from build123d import *

# Parameters (mm, degrees)
F0_W     = 250
F0_H     = 100
F1_DEPTH = 20
F2_W     = 50
F2_H     = 75
F2_W_2   = 44
F2_H_2   = 69
F3_DEPTH = 1200
F4_W     = 50
F4_H     = 75
F4_W_2   = 44
F4_H_2   = 69
F5_DEPTH = 837.2
F6_F1_R  = 1.5
F6_F2_R  = 1.5
F6_F3_R  = 1.5
F6_F4_R  = 1.4999


# Not quite as in the source:
# - a fillet or chamfer is up to 0.001 mm smaller than in the source, because OpenCascade refuses the exact size


with BuildPart() as f1:
    # F0 (on Top) → F1 (new body)
    with BuildSketch(Plane.XY):
        Rectangle(F0_W, F0_H)
    extrude(amount=F1_DEPTH)

    # F2 (on face) → F3 (join)
    with BuildSketch(Plane.XY.offset(20)):
        Rectangle(F2_W, F2_H)
        Rectangle(F2_W_2, F2_H_2, mode=Mode.SUBTRACT)
    extrude(amount=F3_DEPTH)

    # F4 (on face) → F5 (join)
    with BuildSketch(Plane.XZ.offset(37.5)):
        with Locations((0, 1257.5)):
            Rectangle(F4_W, F4_H)
        with Locations((0, 1257.5)):
            Rectangle(F4_W_2, F4_H_2, mode=Mode.SUBTRACT)
    extrude(amount=-F5_DEPTH)

    # F6: fillet of radius 1.5 on 44 edges, made by hand

    # F6_f1
    f6_f1_edges = [f1.edges().sort_by_distance(p)[0] for p in [
        (-22, -34.5, 620),
        (22, 34.5, 620),
        (22, -34.5, 620),
        (-22, 34.5, 620),
        (-22, 381.1, 1292),
        (22, 381.1, 1292),
        (0, 37.5, 1220),
        (22, 381.1, 1223),
        (-22, 381.1, 1223),
        (22, 0, 1220),
        (0, -34.5, 1220),
        (-22, 0, 1220),
        (0, 34.5, 1220),
        (0, 34.5, 20),
        (-22, 0, 20),
        (22, 0, 20),
        (0, -34.5, 20),
    ]]
    fillet(f6_f1_edges, radius=F6_F1_R)

    # F6_f2
    f6_f2_edges = [f1.edges().sort_by_distance(p)[0] for p in [
        (-25, -37.5, 657.5),
        (25, 37.5, 619.25),
        (25, -37.5, 657.5),
        (-25, 37.5, 619.25),
        (25, 381.1, 1295),
        (-25, 381.1, 1295),
        (0, -37.5, 1295),
        (125, -50, 10),
        (-125, -50, 10),
        (125, 50, 10),
        (0, -50, 0),
        (0, -50, 20),
        (0, 50, 20),
        (125, 0, 20),
        (-125, 0, 20),
        (-125, 50, 10),
        (0, 50, 0),
        (125, 0, 0),
        (-125, 0, 0),
        (-25, 37.9393398282, 1219.5606601718),
        (25, 37.9393398282, 1219.5606601718),
    ]]
    fillet(f6_f2_edges, radius=F6_F2_R)

    # F6_f3
    f6_f3_edges = [f1.edges().sort_by_distance(p)[0] for p in [
        (25, 0, 20),
        (-25, 0, 20),
        (0, -37.5, 20),
        (0, 37.5, 20),
        (24.5606601718, 37.0606601718, 20),
        (-24.5606601718, 37.0606601718, 20),
        (-24.5606601718, -37.0606601718, 20),
        (24.5606601718, -37.0606601718, 20),
    ]]
    fillet(f6_f3_edges, radius=F6_F3_R)

    # F6_f4 (radius 1.5 in the source; OpenCascade refuses exactly that, so slightly less here)
    f6_f4_edges = [f1.edges().sort_by_distance(p)[0] for p in [
        (-22, -37.5, 1257.5),
        (0, -37.5, 1223),
        (0, -37.5, 1292),
        (22, -37.5, 1257.5),
        (21.5606601718, -37.5, 1291.5606601718),
        (21.5606601718, -37.5, 1223.4393398282),
        (-21.5606601718, -37.5, 1291.5606601718),
        (-21.5606601718, -37.5, 1223.4393398282),
    ]]
    fillet(f6_f4_edges, radius=F6_F4_R)


solid = f1.part
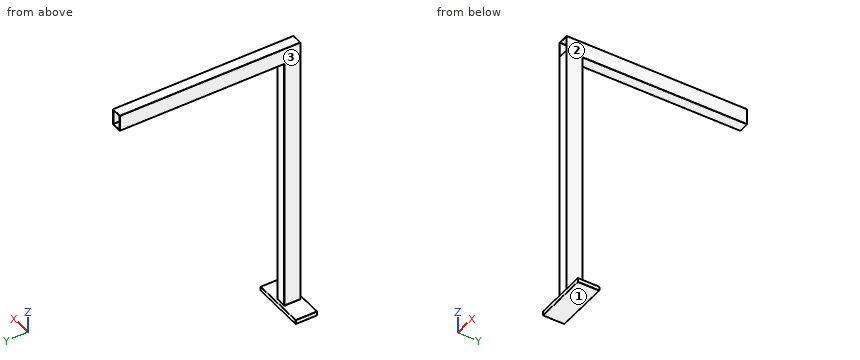
Check sheet for the modelled part. Datum: model origin and axes. Units: mm. Face numbers are marked on the shaded views. A direction names the side the tool comes from. Round coordinates to 2 decimals unless told otherwise and drop trailing zeros. Loops run counter-clockwise (first coordinate to the right, second up) from the corner with the lowest first, then second, coordinate; pieces in that order, holes last. Notation, with made-up numbers: M 74,55 L 129,55 A33 cw 129,91 Z; hole C -7,-8 d8. An arc over 180 degrees is marked long. One line per item, written item: value.
(1) Sectioned sample at A-A, the plane z = 143. Record the cut outline in (x, y), then the cut area to 3 significant figures.
Computed values:
outline: M -25,-36 A1.5 ccw -23.5,-37.5 L 23.5,-37.5 A1.5 ccw 25,-36 L 25,36 A1.5 ccw 23.5,37.5 L -23.5,37.5 A1.5 ccw -25,36 Z; hole M -22,-33 A1.5 ccw -20.5,-34.5 L 20.5,-34.5 A1.5 ccw 22,-33 L 22,33 A1.5 ccw 20.5,34.5 L -20.5,34.5 A1.5 ccw -22,33 Z
area: 714 mm^2
(2) Depth check by flat-ended pin: pin 1 Ø12.5 at (x, z) = (-4.5, 853.5) entering from -Y; pin 2 Ø18.5 at (x, z) = (-30.5, 14) entering from +Y; pin 3 Ø1 at (x, y) = (26.5, 239) entering from +Z. Enter the tip coordinate at first touch or a pass-through.
Computed values:
pin 1: stops at y = -37.5
pin 2: stops at y = 50
pin 3: passes through
(3) Sectioned sample at D-D, the plane y = 7.5. Count the separate pieces of the cut face and the enclosed holes in it, then the cut area to 3 significant figures.
Computed values:
separate pieces: 1
enclosed holes: 2
area: 12,900 mm^2
(4) Sectioned sample at B-B, the plane y = 127. Record the cut outline in (x, z), then the cut area to 3 significant figures.
Computed values:
outline: M -25,1221.5 A1.5 ccw -23.5,1220 L 23.5,1220 A1.5 ccw 25,1221.5 L 25,1293.5 A1.5 ccw 23.5,1295 L -23.5,1295 A1.5 ccw -25,1293.5 Z; hole M -22,1224.5 A1.5 ccw -20.5,1223 L 20.5,1223 A1.5 ccw 22,1224.5 L 22,1290.5 A1.5 ccw 20.5,1292 L -20.5,1292 A1.5 ccw -22,1290.5 Z
area: 714 mm^2
(5) Sectioned sample at C-C, the plane x = -89.5. Record the cut outline in (y, z), then the cut area to 3 significant figures.
Computed values:
outline: M -50,1.5 A1.5 ccw -48.5,0 L 48.5,0 A1.5 ccw 50,1.5 L 50,18.5 A1.5 ccw 48.5,20 L -48.5,20 A1.5 ccw -50,18.5 Z
area: 2,000 mm^2
(6) Access from +Z, -Z, +X, -X, +Y, -Y to the whole of each face (thin tool, end or side, straight path). Record for the marked faces 1, 2 and 3.
Computed values:
face 1: -Z, +X, -X, +Y, -Y
face 2: +Z, +X, +Y, -Y
face 3: +Z, -X, +Y, -Y
(7) Thickness scan on line 1 (Z direction, x = -19.5, y = 91); line 2 (Y direction, x = -23, z = 518.5); line 3 (Y direction, x = 15.5, z = 806.5). Record the ranges inside material, lowest first.
Computed values:
line 1: z = 1220 to 1223, 1292 to 1295
line 2: y = -37.5 to 37.5
line 3: y = -37.5 to -34.5, 34.5 to 37.5
